```python
from build123d import *

# Parameters (mm, degrees)
PAD_DEPTH         = 40
SKETCH002_R       = 4
POCKET_DEPTH      = 5
POCKET_DEPTH_BACK = -5


with BuildPart() as part:
    # Sketch → Pad (new body, symmetric)
    with BuildSketch(Plane.XY):
        Polygon((20, 0), (560, 0), (302.361985, 354.5), (560, 709), (580, 709), (580, 712), (0, 712), (0, 709), (20, 709), (277.638015, 354.5), align=None)
        Polygon((44.723969, 709), (290, 371.509615), (535.276031, 709), align=None, mode=Mode.SUBTRACT)
    extrude(amount=PAD_DEPTH, both=True)

    # Sketch002 → Pocket (cut, two sides)
    with BuildSketch(Plane.XZ.offset(-710)) as pocket_sk:
        with Locations((8, 28)):
            Circle(SKETCH002_R)
        with Locations((290, 28)):
            Circle(SKETCH002_R)
        with Locations((572, 28)):
            Circle(SKETCH002_R)
        with Locations((572, -28)):
            Circle(SKETCH002_R)
        with Locations((290, -28)):
            Circle(SKETCH002_R)
        with Locations((8, -28)):
            Circle(SKETCH002_R)
    extrude(amount=-POCKET_DEPTH, mode=Mode.SUBTRACT)
    extrude(pocket_sk.sketch, amount=-POCKET_DEPTH_BACK, mode=Mode.SUBTRACT)


solid = part.part
```
For this review, take the finished solid that the model builds, in its own axes (mm). A direction names the side the tool comes from. Coordinates: 2 decimals unless noted, no trailing zeros. Loops run counter-clockwise (first coordinate to the right, second up) from the corner with the lowest first, then second, coordinate; pieces in that order, holes last.
1. Insertion check: P1, Ø2, axis at y = 297.5, z = 1, coming from the -X side; P2, Ø10.5, axis at x = 572, z = 28, coming from the -Y side; P3, Ø6, axis at y = 94.5, z = 16, coming from the -X side; P4, Ø6.5, axis at x = 572, z = -28, coming from the +Y side. Each pin has a flat end and moves straight along its axis. Give the tip position at first contact, or say it passes through.
2. For faces 1 (the flat face through (10, 709, 1)), 2 (the flat face through (293, 709, 1)), 3 (the flat face through (429.4, 529.3, 0.6)), 4 (the flat face through (570, 709, 1)), 5 (the flat face through (150.6, 179.7, 0.6)), list the 3-axis set-ups (+Z, -Z, +X, -X, +Y, -Y) from which the entire face can be reached by the end or side of a thin tool; tool diameter is ignored.
3. Add section C-C, the plane y = 405.5. Give the boundary of the cut face in (x, z).
4. Add section B-B, the plane x = 127.5. Give the boundary of the cut face in (y, z), then the cut area to 3 significant figures.
5. Add section D-D, the plane x = 458.5. Give the boundary of the cut face in (y, z), then the cut area to 3 significant figures.
6. Mouldability with a two-part tool opening along X and no side actions: class faces 6 (the flat face through (165.645, 542.617, 0.56)), 7 (the flat face through (286, 0, 1)), 8 (the flat face through (147.016, 534.232, 0.56)) as +X half, -X half, draft (parallel to the pull), parting line (faces both ways), or undercut.
7. Add section A-A, the plane z = -9. Give the boundary of the cut face in (x, y).
8. For line 1 (Z direction, x = 290, y = 710.95); line 2 (X direction, y = 709.5, z = -28); line 3 (Y direction, x = 127.5, z = 4.5), list the stretches that pass through material, from the lowest coordinate up.
Result:
1. P1: stops at x = 235.49
1. P2: stops at y = 709
1. P3: stops at x = 86.5
1. P4: passes through
2. face 1: +Z, -Z, -X, -Y
2. face 2: +Z, -Z
2. face 3: +Z, -Z, +X
2. face 4: +Z, -Z, +X, -Y
2. face 5: +Z, -Z, -X
3. outline: (240.57, -40) - (265.3, -40) - (265.3, 40) - (240.57, 40) - close; (314.7, -40) - (339.43, -40) - (339.43, 40) - (314.7, 40) - close
4. outline: (0, -40) - (147.92, -40) - (147.92, 40) - (0, 40) - close; (561.08, -40) - (595.1, -40) - (595.1, 40) - (561.08, 40) - close; (709, -40) - (712, -40) - (712, 40) - (709, 40) - close
4. area: 14,800 mm2
5. outline: (0, -40) - (139.66, -40) - (139.66, 40) - (0, 40) - close; (569.34, -40) - (603.36, -40) - (603.36, 40) - (569.34, 40) - close; (709, -40) - (712, -40) - (712, 40) - (709, 40) - close
5. area: 14,100 mm2
6. face 6: undercut
6. face 7: draft
6. face 8: -X half
7. outline: (0, 709) - (20, 709) - (277.64, 354.5) - (20, 0) - (560, 0) - (302.36, 354.5) - (560, 709) - (580, 709) - (580, 712) - (0, 712) - close; hole (44.72, 709) - (290, 371.51) - (535.28, 709) - close
8. line 1: z = -40 to -32, -24 to 24, 32 to 40
8. line 2: x = 0 to 4, 12 to 286, 294 to 568, 576 to 580
8. line 3: y = 0 to 147.92, 561.08 to 595.1, 709 to 712
